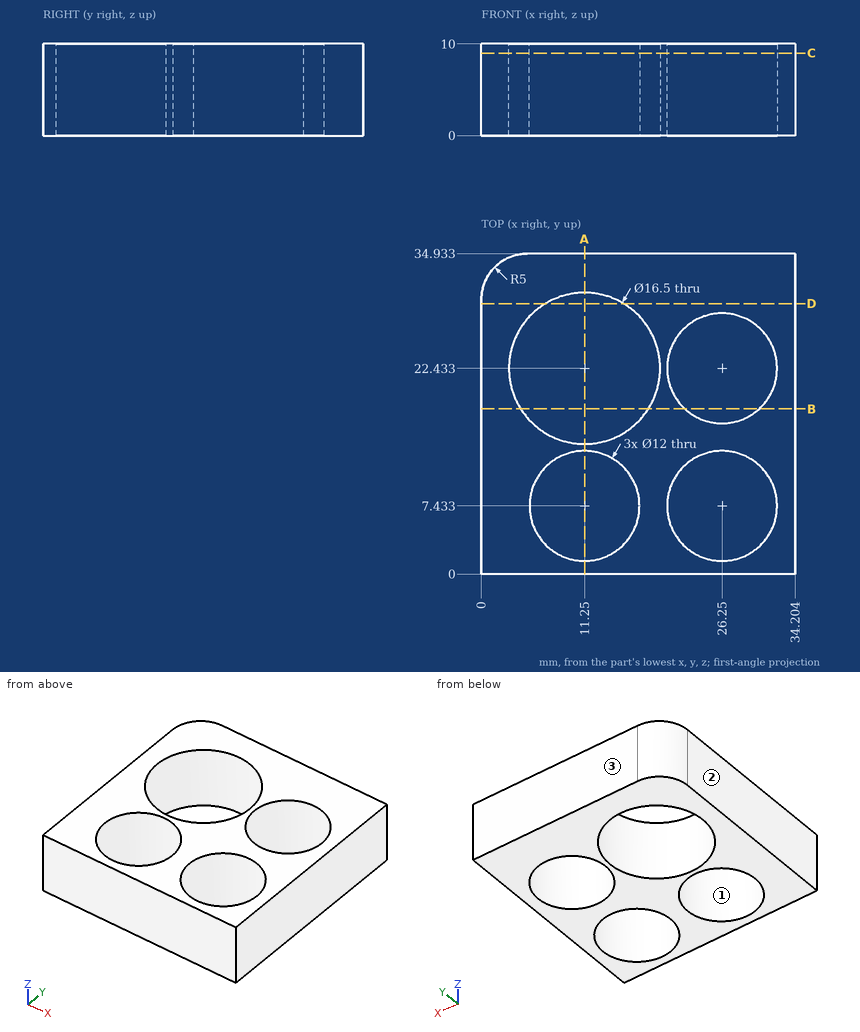
Can you work these out from the drawing? Everything is in mm from the part's minimum corner. Round coordinates to 2 decimals unless told otherwise and drop trailing zeros. Loops run counter-clockwise (first coordinate to the right, second up) from the corner with the lowest first, then second, coordinate; pieces in that order, holes last. Notation, with made-up numbers: M -38,11 L -18,11 A27 ccw -18,47 Z; hole C 17.5,-25 d5. An arc over 180 degrees is marked long. Write item = value, one per line.
1. Thinking about a two-plate mould opening in X: for the marked faces 1, 2 and 3, which applies, +X half, -X half, draft (parallel to the pull), parting line (faces both ways), or undercut?
Results below:
face_1 = undercut
face_2 = -X half
face_3 = draft
2. I want a section at C-C, the plane z = 9. Write out the boundary of the cut face in (x, y).
Results below:
outline = M 0,0 L 34.2,0 L 34.2,34.93 L 5,34.93 A5 ccw 0,29.93 Z; hole C 11.25,22.43 d16.5; hole C 11.25,7.43 d12; hole C 26.25,7.43 d12; hole C 26.25,22.43 d12
3. Will this pin go through, and if not, where does the flat tip stop? P1, Ø4, axis at y = 29, z = 4, coming from the -X side.
Results below:
P1 = 0
4. I need wall thicknesses on probe 1 along Y at (x, z) = (26.25, 3); probe 2 along Y at (x, z) = (11.25, 4); probe 3 along X at (y, z) = (12, 3.75). Which ranges of each line are inside material? Lowest first, please.
Results below:
probe_1 = 0 to 1.43, 13.43 to 16.43, 28.43 to 34.93
probe_2 = 0 to 1.43, 13.43 to 14.18, 30.68 to 34.93
probe_3 = 0 to 7.36, 15.14 to 22.36, 30.14 to 34.2
5. I want a section at A-A, the plane x = 11.25. Write out the boundary of the cut face in (y, z).
Results below:
outline = M 0,0 L 1.43,0 L 1.43,10 L 0,10 Z; M 13.43,0 L 14.18,0 L 14.18,10 L 13.43,10 Z; M 30.68,0 L 34.93,0 L 34.93,10 L 30.68,10 Z
6. I want a section at B-B, the plane y = 18. Write out the boundary of the cut face in (x, z), and give its area (3 significant figures).
Results below:
outline = M 0,0 L 4.29,0 L 4.29,10 L 0,10 Z; M 18.21,0 L 22.21,0 L 22.21,10 L 18.21,10 Z; M 30.29,0 L 34.2,0 L 34.2,10 L 30.29,10 Z
area = 122 mm²
7. I want a section at D-D, the plane y = 29.5. Write out the boundary of the cut face in (x, z), and give its area (3 significant figures).
Results below:
outline = M 0,0 L 6.99,0 L 6.99,10 L 0,10 Z; M 15.51,0 L 34.2,0 L 34.2,10 L 15.51,10 Z
area = 257 mm²
